Autodesk Inventor part; units mm, degrees
ref_plane "YZ Plane" through (0, 0, 0) normal (1, 0, 0) x (0, 1, 0)
ref_plane "XZ Plane" through (0, 0, 0) normal (0, 1, 0) x (-1, 0, 0)
ref_plane "XY Plane" through (0, 0, 0) normal (0, 0, 1) x (1, 0, 0)
sketch "Sketch2" plane through (0, 0, 0) normal (0, 0, 1) x (1, 0, 0)
  line L0 (-21, 0) -> (21, 0) construction
  line L1 (0, -21) -> (0, 21) construction
  circle A0 centre (0, 0) radius 15
  dimension "d0" = 30
extrude "Extrusion1" add sketch "Sketch2" along normal blind 5
sketch "Sketch3" plane through (0, 0, 5) normal (0, 0, 1) x (1, 0, 0)
  line L0 (-21, 0) -> (21, 0) construction
  line L1 (0, -21) -> (0, 21) construction
  line L2 (-2, 7.5) -> (2, 7.5)
  line L3 (2, 7.5) -> (2, -7.5)
  line L4 (2, -7.5) -> (-2, -7.5)
  line L5 (-2, -7.5) -> (-2, 7.5)
  point P0 (0, 0)
  dimension "d3" = 2
  dimension "d5" = 15
extrude "Extrusion2" add sketch "Sketch3" along normal blind 30
sketch "Sketch4" plane through (0, 0, 5) normal (0, 0, 1) x (1, 0, 0)
  circle A0 centre (0, 0) radius 15 construction
  line L0 (0, -21) -> (0, 21) construction
  line L1 (-21, 0) -> (21, 0) construction
  circle A1 centre (0, 0) radius 14
  circle A2 centre (0, 0) radius 15
  dimension "d8" = 28
extrude "Extrusion3" add sketch "Sketch4" along normal blind 5
properties part number "P011_Chapeau_chambre"
CAD build for the part. Positions are in the model's coordinates, mm. A direction names the side the tool comes from. Give positions to 0.01 mm unless a question says otherwise; leave off trailing zeros. Write each loop counter-clockwise with the first axis right and the second up, starting at its lowest first coordinate (ties: lowest second). Pieces come first, ordered by that corner, then holes. Notation, with made-up numbers: (56, 81.25) - (71, 81.25) arc R15 ccw to (71, 95.25) - close; hole circle Ø10 at (42.25, -32.5). An arc over 180 degrees is marked (long way). Put each result on its own line as item: value.
(1) Saw through at C-C (x = 0). List the corners of the cut face in (y, z).
Working result:
outline: (-15, 0) - (15, 0) - (15, 10) - (14, 10) - (14, 5) - (7.5, 5) - (7.5, 35) - (-7.5, 35) - (-7.5, 5) - (-14, 5) - (-14, 10) - (-15, 10) - close
(2) Saw through at D-D (z = 3.5). List the corners of the cut face in (x, y).
Working result:
outline: circle Ø30 at (0, 0)
(3) Saw through at B-B (y = 0). List the corners of the cut face in (x, z).
Working result:
outline: (-15, 0) - (15, 0) - (15, 10) - (14, 10) - (14, 5) - (2, 5) - (2, 35) - (-2, 35) - (-2, 5) - (-14, 5) - (-14, 10) - (-15, 10) - close
(4) Tool access for faces 4 (the flat face through (0, 0, 35)), 5 (the flat face through (0, -7.5, 20)): list every direction of +Z, -Z, +X, -X, +Y, -Y with a clear straight run to the whole face (end or side of a thin tool).
Working result:
face 4: +Z, +X, -X, +Y, -Y
face 5: +Z
(5) Saw through at A-A (z = 8.5). List the corners of the cut face in (x, y), then the cut area to 3 significant figures.
Working result:
outline: circle Ø30 at (0, 0); (-2, -7.5) - (2, -7.5) - (2, 7.5) - (-2, 7.5) - close; hole circle Ø28 at (0, 0)
area: 151 mm^2
(6) Pull direction X, two halves, no side cores. Call faces 1 (the flat face through (0, 0, 0)), 2 (the cylindrical face through (12.932, 5.362, 7.465)), 3 (the cylindrical face through (-14.985, -0.66, 4.93)): released by +X, released by -X, zero draft, split by the parting line, or undercut.
Working result:
face 1: zero draft
face 2: undercut
face 3: split by the parting line
(7) Drop flat-ended pins along their axis: pin 1 Ø5 at (x, y) = (0, 9.5) entering from +Z; pin 2 Ø4.5 at (y, z) = (-0.5, 23.5) entering from +X; pin 3 Ø1.5 at (x, z) = (-2, 13.5) entering from -Y; pin 4 Ø7.5 at (y, z) = (-2.5, 22.5) entering from -X. Give the stop position or say it passes through.
Working result:
pin 1: z = 35
pin 2: x = 2
pin 3: y = -7.5
pin 4: x = -2
(8) Wall check: L1, parallel to Y at x = 0, z = 6.4; L2, parallel to X at y = 4, z = 5.5; L3, parallel to X at y = -3, z = 9. Give the ranges that are in metal, low to high.
Working result:
L1: -15 to -14, -7.5 to 7.5, 14 to 15
L2: -14.46 to -13.42, -2 to 2, 13.42 to 14.46
L3: -14.7 to -13.67, -2 to 2, 13.67 to 14.7
